from build123d import *

# Parameters (mm, degrees)
EXTRUDE_1_DEPTH          = 6.5
EXTRUDE_START            = 9
EXTRUDE_2_DEPTH          = 9
PATTERN_CIRCULAR_1_COUNT = 2
PATTERN_CIRCULAR_1_ANGLE = 6
CUT_EXTRUDE_2_DEPTH      = 1.75
FILLET_1_R               = 1
CHAMFER_1_SIZE           = 1
FILLET_2_R               = 0.5


with BuildPart() as part:
    # Эскиз1 → Бобышка-Вытянуть1 (new, symmetric)
    with BuildSketch(Plane.XY):
        with BuildLine():
            Line((14.283525476, 45.301555161), (15.486348674, 49.116422964))
            ThreePointArc((15.486348674, 49.116422964), (9.314199823, 50.65072242), (3, 51.412547107))
            Line((3, 51.412547107), (3, 54.918120871))
            ThreePointArc((3, 54.918120871), (0, 55), (-3, 54.918120871))
            Line((-3, 54.918120871), (-3, 51.412547107))
            ThreePointArc((-3, 51.412547107), (-9.314199823, 50.65072242), (-15.486348674, 49.116422964))
            Line((-15.486348674, 49.116422964), (-14.283525476, 45.301555161))
            ThreePointArc((-14.283525476, 45.301555161), (0, 47.5), (14.283525476, 45.301555161))
        make_face()
    extrude(amount=EXTRUDE_1_DEPTH, both=True)

    # Эскиз2 → Бобышка-Вытянуть2 (add)
    with BuildSketch(Plane.XY.offset(6.5).offset(EXTRUDE_START)):
        with BuildLine():
            Line((3, 52.915026221), (3, 54.918120871))
            ThreePointArc((3, 54.918120871), (0, 55), (-3, 54.918120871))
            Line((-3, 54.918120871), (-3, 52.915026221))
            ThreePointArc((-3, 52.915026221), (0, 53), (3, 52.915026221))
        make_face()
    extrude(amount=-EXTRUDE_2_DEPTH)

    # Эскиз4 → Вырез-Повернуть1 (revolve, cut)
    with BuildSketch(Plane.XY):
        Polygon((15.202210874, 58.068539542), (10.703189787, 38.581138246), (8.998042174, 38.974802591), (13.497063261, 58.462203887), align=None)
    cut_revolve_1 = revolve(axis=Axis((0, 0, 0), (0.22495105434386545, 0.9743700647852351, 0)), mode=Mode.SUBTRACT)

    # Круговой массив1: Вырез-Повернуть1 ×2 about axis
    pattern_circular_1_axis = Axis((0, 0, 6.5), (0, 0, 1))
    for i in range(1, PATTERN_CIRCULAR_1_COUNT):
        add(cut_revolve_1.rotate(pattern_circular_1_axis, i * PATTERN_CIRCULAR_1_ANGLE / (PATTERN_CIRCULAR_1_COUNT - 1)), mode=Mode.SUBTRACT)

    # Эскиз6 → Вырез-Вытянуть2 (cut, symmetric)
    with BuildSketch(Plane.XY):
        with BuildLine():
            Line((5.788793812, 47.145942203), (6.276271185, 51.11612681))
            ThreePointArc((6.276271185, 51.11612681), (8.94288115, 50.71759928), (11.584979299, 50.180058336))
            Line((11.584979299, 50.180058336), (10.685175081, 46.282578077))
            ThreePointArc((10.685175081, 46.282578077), (8.248288439, 46.778368268), (5.788793812, 47.145942203))
        make_face()
    cut_extrude_2 = extrude(amount=CUT_EXTRUDE_2_DEPTH, both=True, mode=Mode.SUBTRACT)

    # Зеркальное отражение1: Вырез-Повернуть1, Вырез-Вытянуть2 across plane
    add(cut_revolve_1.mirror(Plane(origin=(0, 0, 0), x_dir=(0, 0, 1), z_dir=(1, 0, 0))), mode=Mode.SUBTRACT)
    add(cut_extrude_2.mirror(Plane(origin=(0, 0, 0), x_dir=(0, 0, 1), z_dir=(1, 0, 0))), mode=Mode.SUBTRACT)

    # Зеркальное отражение1 copy 1 sketch → Зеркальное отражение1 copy 1 (revolve, cut)
    with BuildSketch(Plane(origin=(0, 0, 0), x_dir=(-0.9945218953682733, 0.10452846326765369, 0), z_dir=(0, 0, 1))):
        Polygon((15.202210874, -58.068539542), (10.703189787, -38.581138246), (8.998042174, -38.974802591), (13.497063261, -58.462203887), align=None)
    revolve(axis=Axis((0, 0, 0), (0.12186934340514771, -0.992546151641322, 0)), mode=Mode.SUBTRACT)

    # Скругление1
    fillet_1_edges = [part.edges().sort_by_distance(p)[0] for p in [
        (-3, 51.412547107, 0),
        (3, 51.412547107, 0),
    ]]
    fillet(fillet_1_edges, radius=FILLET_1_R)

    # Фаска1
    chamfer_1_edges = [part.edges().sort_by_distance(p)[0] for p in [
        (14.884937075, 47.208989062, -6.5),
        (-14.884937075, 47.208989062, 6.5),
        (-14.884937075, 47.208989062, -6.5),
        (14.884937075, 47.208989062, 6.5),
    ]]
    chamfer(chamfer_1_edges, length=CHAMFER_1_SIZE)

    # Скругление2
    fillet_2_edges = [part.edges().sort_by_distance(p)[0] for p in [
        (-3, 53.916573546, 15.5),
        (3, 53.916573546, 15.5),
    ]]
    fillet(fillet_2_edges, radius=FILLET_2_R)


solid = part.part
Work out the finished part from the listing and answer in its coordinate system (mm). A direction names the side the tool comes from. Give positions to 0.01 mm unless a question says otherwise; leave off trailing zeros. Write each loop counter-clockwise with the first axis right and the second up, starting at its lowest first coordinate (ties: lowest second). Pieces come first, ordered by that corner, then holes.
Q1. A tool of negligible diameter and unlimited length cuts with its end or side. For faces 4 (the face through (3, 54, 4)), 5 (the face through (-3, 54, 4)), 6 (the face through (4.29, 49.3, -0.04)), from which of +Z, -Z, +X, -X, +Y, -Y can it reach the whole face along a straight path? Write none if from no direction.
Answer:
face 4: +Z, -Z, +X, +Y
face 5: +Z, -Z, -X, +Y
face 6: -Y
Q2. For a pull along X with two mould halves and no side action, classify faces 1 (the face through (9, 49, -1.75)), 2 (the face through (-14.422, 47.379, 5.993)), 3 (the face through (14.877, 47.182, 0.077)) as released by +X, released by -X, zero draft, split by the parting line, or undercut.
Answer:
face 1: undercut
face 2: released by -X
face 3: released by +X
Q3. Given pin 1 (1.3 mm diameter, centred on y = 54, z = 5.5, fed in from +X); pin 2 (0.8 mm diameter, centred on y = 54, z = 8, fed in from -X); pin 3 (6 mm diameter, centred on x = -8, z = 11, fed in from -Y); pin 4 (5.5 mm diameter, centred on x = -9.5, y = 48, fed in from +Z), each flat-ended and moving along its own axis, determine where each tip first touches the part or whether it passes through.
Answer:
pin 1: stops at x = 3
pin 2: stops at x = -3
pin 3: passes through
pin 4: stops at z = 6.5
Q4. The part is cut by section A-A on x = -9.5. Give the vertices of the cut face in (y, z).
Answer:
outline: (46.54, -6.5) - (50.62, -6.5) - (50.62, -1.75) - (46.54, -1.75) - close; (46.54, 1.75) - (50.62, 1.75) - (50.62, 6.5) - (46.54, 6.5) - close
Q5. Straight lines are drawn through the part: L1, parallel to X at y = 53.25, z = 8.5; L2, parallel to Z at x = -9, y = 50.5; L3, parallel to Z at x = -3.5, y = 47.5. For each, find the intervals that lie inside material, in ascending order.
Answer:
L1: x = -3 to 3
L2: z = -6.5 to -1.75, 1.75 to 6.5
L3: z = -6.5 to 6.5
Q6. The part is cut by section D-D on x = 9. Give the vertices of the cut face in (y, z), and give its area (3 significant figures).
Answer:
outline: (46.64, -6.5) - (50.71, -6.5) - (50.71, -1.75) - (46.64, -1.75) - close; (46.64, 1.75) - (50.71, 1.75) - (50.71, 6.5) - (46.64, 6.5) - close
area: 38.6 mm2
Q7. The part is cut by section B-B on y = 54. Give the vertices of the cut face in (x, z), and give its area (3 significant figures).
Answer:
outline: (-3, -6.5) - (3, -6.5) - (3, 15) arc R0.5 ccw to (2.5, 15.5) - (-2.5, 15.5) arc R0.5 ccw to (-3, 15) - close
area: 132 mm2
Q8. The part is cut by section C-C on z = 5. Give the vertices of the cut face in (x, y), and give its area (3 significant figures).
Answer:
outline: (-15.49, 49.12) - (-14.28, 45.3) arc R47.5 cw to (14.28, 45.3) - (15.49, 49.12) arc R51.5 ccw to (3.92, 51.35) arc R1 cw to (3, 52.35) - (3, 54.92) arc R55 ccw to (-3, 54.92) - (-3, 52.35) arc R1 cw to (-3.92, 51.35) arc R51.5 ccw to start
area: 142 mm2
